The listing builds one solid part. Answer for the finished solid, in the listing's coordinates (mm). A direction names the side the tool comes from. Round coordinates to 2 decimals unless told otherwise and drop trailing zeros. Loops run counter-clockwise (first coordinate to the right, second up) from the corner with the lowest first, then second, coordinate; pieces in that order, holes last. Notation, with made-up numbers: (50.5, -3.75) -> (82.5, -3.75) arc R5 cw to (82.5, 3.25) -> close; hole circle Ø2 at (25.5, -8). An arc over 180 degrees is marked (long way). One line per question, with ' | ' between items.
from build123d import *

# Parameters (mm, degrees)
BOSS_EXTRUDE1_DEPTH = 20
SKETCH2_R           = 1.7
CUT_EXTRUDE1_DEPTH  = 40
CHAMFER1_SIZE       = 2
FILLET1_R           = 10


with BuildPart() as part:
    # Sketch1 → Boss-Extrude1 (new, symmetric)
    with BuildSketch(Plane.XY):
        Polygon((0, 0), (13, 0), (13, 3), (3, 3), (3, 80), (0, 80), align=None)
    extrude(amount=BOSS_EXTRUDE1_DEPTH, both=True)

    # Sketch2 → Cut-Extrude1 (cut)
    with BuildSketch(Plane(origin=(0, 3, 0), x_dir=(1, 0, 0), z_dir=(0, 1, 0))):
        with Locations(Location((8, 15, 0), (0, 0, 180))):
            Circle(SKETCH2_R)
        with Locations(Location((8, -15, 0), (0, 0, 180))):
            Circle(SKETCH2_R)
    extrude(amount=-CUT_EXTRUDE1_DEPTH, mode=Mode.SUBTRACT)

    # Chamfer1
    chamfer1_edges = [part.edges().sort_by_distance(p)[0] for p in [
        (3, 3, 0),
    ]]
    chamfer(chamfer1_edges, length=CHAMFER1_SIZE)

    # Fillet1
    fillet1_edges = [part.edges().sort_by_distance(p)[0] for p in [
        (1.5, 80, 20),
        (1.5, 80, -20),
    ]]
    fillet(fillet1_edges, radius=FILLET1_R)


solid = part.part
Q1. Find the intervals of material crossed by line 1 (Z direction, x = 8, y = 0.75); line 2 (Y direction, x = 12.5, z = 7), in increasing order. Write a range as from..to.
Numbers:
line 1: -20..-16.7, -13.3..13.3, 16.7..20 | line 2: 0..3
Q2. A cutting plane is placed at D-D on y = 26.5. Give the vertices of the cut face in (x, z).
Numbers:
outline: (0, -20) -> (3, -20) -> (3, 20) -> (0, 20) -> close
Q3. Given pin 1 Ø5 at (y, z) = (22.5, 11.5) entering from +X; pin 2 Ø3 at (x, z) = (8, -15) entering from -Y; pin 3 Ø4 at (x, z) = (8, 15) entering from +Y, each flat-ended and moving along its own axis, determine where each tip first touches the part or whether it passes through.
Numbers:
pin 1: x = 3 | pin 2: through | pin 3: y = 3
Q4. A cutting plane is placed at B-B on z = 15. Give the vertices of the cut face in (x, y), plus the area to 3 significant figures.
Numbers:
outline: (0, 0) -> (6.3, 0) -> (6.3, 3) -> (5, 3) -> (3, 5) -> (3, 78.66) -> (0, 78.66) -> close; (9.7, 0) -> (13, 0) -> (13, 3) -> (9.7, 3) -> close | area: 258 mm^2
Q5. A cutting plane is placed at A-A on x = 8. Give the vertices of the cut face in (y, z), plus the area to 3 significant figures.
Numbers:
outline: (0, -20) -> (3, -20) -> (3, -16.7) -> (0, -16.7) -> close; (0, -13.3) -> (3, -13.3) -> (3, 13.3) -> (0, 13.3) -> close; (0, 16.7) -> (3, 16.7) -> (3, 20) -> (0, 20) -> close | area: 99.6 mm^2
Q6. For a pull along Z with two mould halves and no side action, classify faces 1 (the face through (9, 3, 0)), 2 (the face through (2, 33, -20)), 3 (the face through (9.7, 1.52, -14.93)) as pulls with the +Z half, pulls with the -Z half, needs draft (parallel to the pull), parting line crosses it, or undercut.
Numbers:
face 1: needs draft | face 2: pulls with the -Z half | face 3: undercut
Q7. A cutting plane is placed at C-C on z = 8. Give the vertices of the cut face in (x, y), plus the area to 3 significant figures.
Numbers:
outline: (0, 0) -> (13, 0) -> (13, 3) -> (5, 3) -> (3, 5) -> (3, 80) -> (0, 80) -> close | area: 272 mm^2
Q8. For faces 4 (the face through (2, 33, 20)), 5 (the face through (3, 42, 0)), determine the directions among +Z, -Z, +X, -X, +Y, -Y from which every point of the face is accessible in a straight line to the end or side of a thin tool.
Numbers:
face 4: +Z, +X, -X, +Y, -Y | face 5: +Z, -Z, +X, +Y
